Read the model definition and answer for the solid it produces. Units are mm, in the model's axes. Face numbers are marked on the shaded views. A direction names the side the tool comes from. Give positions to 0.01 mm unless a question says otherwise; leave off trailing zeros. Loops run counter-clockwise (first coordinate to the right, second up) from the corner with the lowest first, then second, coordinate; pieces in that order, holes last. Notation, with made-up numbers: (2.5, -21.5) - (14.5, -21.5) arc R23 ccw to (14.5, 7.5) - close; hole circle Ø5 at (1, 8). An arc over 180 degrees is marked (long way). Write item = value, one per line.
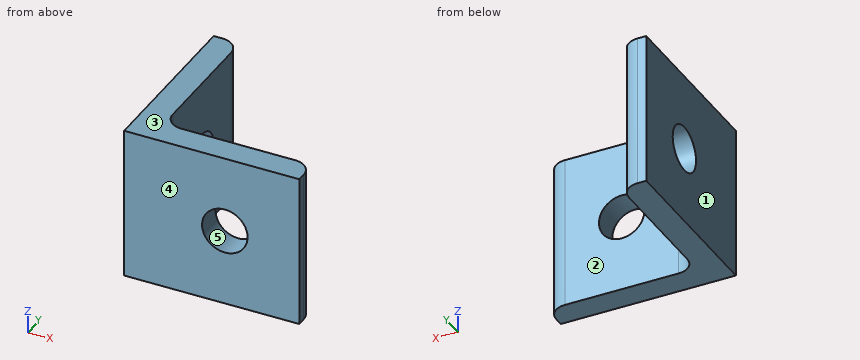
```python
from build123d import *

# Parameters (mm, degrees)
BOSS_EXTRUDE1_DEPTH = 22.225
SKETCH2_R           = 3.302
CUT_EXTRUDE1_DEPTH  = 38.765153581
SKETCH3_R           = 3.302
CUT_EXTRUDE2_DEPTH  = 38.765153581
FILLET1_R           = 2.54


with BuildPart() as part:
    # Sketch1 → Boss-Extrude1 (new body)
    with BuildSketch(Plane.XY):
        Polygon((0, 21.59), (0, 0), (21.59, 0), (21.59, -3.81), (-3.81, -3.81), (-3.81, 21.59), align=None)
    extrude(amount=BOSS_EXTRUDE1_DEPTH)

    # Sketch2 → Cut-Extrude1 (cut, through all)
    with BuildSketch(Plane(origin=(0, 0, 0), x_dir=(1, 0, 0), z_dir=(0, 1, 0))):
        with Locations(Location((10.795, -11.1125, 0), (0, 0, 270))):
            Circle(SKETCH2_R)
    extrude(amount=-CUT_EXTRUDE1_DEPTH, mode=Mode.SUBTRACT)

    # Sketch3 → Cut-Extrude2 (cut, through all)
    with BuildSketch(Plane(origin=(0, 0, 0), x_dir=(0, 0, -1), z_dir=(1, 0, 0))):
        with Locations(Location((-11.1125, 10.795, 0), (0, 0, 90))):
            Circle(SKETCH3_R)
    extrude(amount=-CUT_EXTRUDE2_DEPTH, mode=Mode.SUBTRACT)

    # Fillet1
    fillet1_edges = [part.edges().sort_by_distance(p)[0] for p in [
        (0, 21.59, 11.1125),
        (0, 0, 11.1125),
        (21.59, 0, 11.1125),
    ]]
    fillet(fillet1_edges, radius=FILLET1_R)


solid = part.part
```
1) Each of these flat-tipped pins is pushed along its axis until it touches: P1, Ø3, axis at y = 4.5, z = 10.5, coming from the +X side; P2, Ø8, axis at y = 6, z = 15, coming from the +X side; P3, Ø5, axis at x = 14, z = 10, coming from the +Y side; P4, Ø1.5, axis at y = 11.5, z = 10, coming from the +X side. Where does it stop, or does it pass through?
Output:
P1 = 0
P2 = 0.06
P3 = 0
P4 = through
2) The mould has two halves that part along Z. Classify the marked faces 3, 4 and 5: pulls with the +Z half, pulls with the -Z half, needs draft (parallel to the pull), parting line crosses it, or undercut.
Output:
face_3 = pulls with the +Z half
face_4 = needs draft
face_5 = undercut
3) A cutting plane is placed at A-A on y = 9.75. Determine the outline of the cut face in (x, z) (3 decimals).
Output:
outline = (-3.81, 0) - (0, 0) - (0, 7.98) - (-3.81, 7.98) - close; (-3.81, 14.245) - (0, 14.245) - (0, 22.225) - (-3.81, 22.225) - close
4) A cutting plane is placed at D-D on x = 15. Determine the outline of the cut face in (y, z) (3 decimals), then the cut area to 3 significant figures.
Output:
outline = (-3.81, 0) - (0, 0) - (0, 22.225) - (-3.81, 22.225) - close
area = 84.7 mm²
5) A cutting plane is placed at C-C on z = 6.25. Determine the outline of the cut face in (x, y), then the cut area to 3 significant figures.
Output:
outline = (-3.81, -3.81) - (21.59, -3.81) - (21.59, -2.54) arc R2.54 ccw to (19.05, 0) - (2.54, 0) arc R2.54 cw to (0, 2.54) - (0, 19.05) arc R2.54 ccw to (-2.54, 21.59) - (-3.81, 21.59) - close
area = 178 mm²
6) A tool of negligible diameter and unlimited length cuts with its end or side. For the marked faces 1 and 2, from which of +Z, -Z, +X, -X, +Y, -Y can it reach the whole face along a straight path? Write none if from no direction.
Output:
face_1 = +Z, -Z, -X, +Y, -Y
face_2 = +Z, -Z, +X, +Y
7) A cutting plane is placed at B-B on x = 9.5. Determine the outline of the cut face in (y, z) (3 decimals).
Output:
outline = (-3.81, 0) - (0, 0) - (0, 8.075) - (-3.81, 8.075) - close; (-3.81, 14.15) - (0, 14.15) - (0, 22.225) - (-3.81, 22.225) - close
8) Find the intervals of material crossed by probe 1 along Z at (x, y) = (-2.25, 11) (3 decimals); probe 2 along Y at (x, z) = (17.5, 19.75); probe 3 along Z at (x, y) = (8, -1.5) (3 decimals), in increasing order.
Output:
probe_1 = 0 to 7.817, 14.408 to 22.225
probe_2 = -3.81 to 0
probe_3 = 0 to 9.354, 12.871 to 22.225
